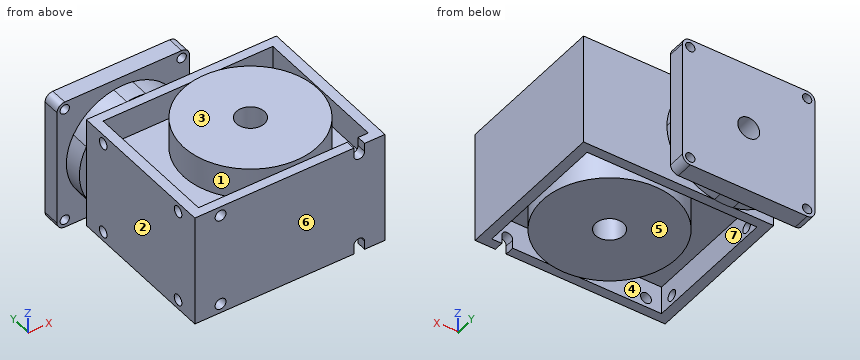
```python
from build123d import *

# Parameters (mm, degrees)
CROQUIS2_W              = 122
CROQUIS2_H              = 72
SALIENTE_EXTRUIR1_DEPTH = 100
CROQUIS3_W              = 109
CROQUIS3_H              = 88
CORTAR_EXTRUIR1_DEPTH   = 18
CROQUIS4_W              = 109
CROQUIS4_H              = 88
CORTAR_EXTRUIR2_DEPTH   = 18
SALIENTE_EXTRUIR2_DEPTH = 12
CROQUIS6_W              = 85
CROQUIS6_H              = 85
SALIENTE_EXTRUIR3_DEPTH = 11
CROQUIS7_R              = 43
SALIENTE_EXTRUIR7_DEPTH = 20
SALIENTE_EXTRUIR8_START = 20
CROQUIS8_R              = 43
SALIENTE_EXTRUIR8_DEPTH = 20
CROQUIS9_R              = 9
CORTAR_EXTRUIR3_DEPTH   = 76
CROQUIS10_R             = 3.5
CORTAR_EXTRUIR5_DEPTH   = 6
CROQUIS11_R             = 3.5
CORTAR_EXTRUIR6_DEPTH   = 6.5
CROQUIS12_R             = 7
CORTAR_EXTRUIR7_DEPTH   = 36
CROQUIS13_R             = 3
CORTAR_EXTRUIR8_DEPTH   = 11
REDONDEO2_R             = 5


with BuildPart() as part:
    # Croquis2 → Saliente-Extruir1 (new body)
    with BuildSketch(Plane(origin=(0, 0, 0), x_dir=(1, 0, 0), z_dir=(0, 1, 0))):
        Rectangle(CROQUIS2_W, CROQUIS2_H)
    extrude(amount=SALIENTE_EXTRUIR1_DEPTH)

    # Croquis3 → Cortar-Extruir1 (cut)
    with BuildSketch(Plane(origin=(0, 0, -36), x_dir=(-1, 0, 0), z_dir=(0, 0, -1))):
        with Locations((0, 50)):
            Rectangle(CROQUIS3_W, CROQUIS3_H)
    extrude(amount=-CORTAR_EXTRUIR1_DEPTH, mode=Mode.SUBTRACT)

    # Croquis4 → Cortar-Extruir2 (cut)
    with BuildSketch(Plane.XY.offset(36)):
        with Locations((0, 50)):
            Rectangle(CROQUIS4_W, CROQUIS4_H)
    extrude(amount=-CORTAR_EXTRUIR2_DEPTH, mode=Mode.SUBTRACT)

    # Croquis5 → Saliente-Extruir2 (add)
    with BuildSketch(Plane(origin=(0, 100, 0), x_dir=(1, 0, 0), z_dir=(0, 1, 0))):
        with BuildLine():
            Line((-61, 17.557049866), (-61, 0))
            Line((-61, 0), (-29, 0))
            Line((-29, 0), (7.5, 0))
            ThreePointArc((7.5, 0), (-1.143141768, 23.584856359), (-22.979202711, 36))
            Line((-22.979202711, 36), (-35.020797289, 36))
            ThreePointArc((-35.020797289, 36), (-50.128910503, 29.762713938), (-61, 17.557049866))
        make_face()
        with BuildLine():
            Line((-61, -17.557049866), (-61, 0))
            Line((-61, 0), (-61, 17.557049866))
            ThreePointArc((-61, 17.557049866), (-65.5, 0), (-61, -17.557049866))
        make_face()
        with BuildLine():
            Line((-29, 0), (-61, 0))
            Line((-61, 0), (-61, -17.557049866))
            ThreePointArc((-61, -17.557049866), (-50.128910503, -29.762713938), (-35.020797289, -36))
            Line((-35.020797289, -36), (-22.979202711, -36))
            ThreePointArc((-22.979202711, -36), (-1.143141768, -23.584856359), (7.5, 0))
            Line((7.5, 0), (-29, 0))
        make_face()
        with BuildLine():
            Line((-22.979202711, -36), (-35.020797289, -36))
            ThreePointArc((-35.020797289, -36), (-29, -36.5), (-22.979202711, -36))
        make_face()
        with BuildLine():
            ThreePointArc((-22.979202711, 36), (-29, 36.5), (-35.020797289, 36))
            Line((-35.020797289, 36), (-22.979202711, 36))
        make_face()
    extrude(amount=SALIENTE_EXTRUIR2_DEPTH)

    # Croquis6 → Saliente-Extruir3 (add)
    with BuildSketch(Plane(origin=(0, 112, 0), x_dir=(1, 0, 0), z_dir=(0, 1, 0))):
        with Locations((-29, 0)):
            Rectangle(CROQUIS6_W, CROQUIS6_H)
    extrude(amount=SALIENTE_EXTRUIR3_DEPTH)

    # Croquis7 → Saliente-Extruir7 (add)
    with BuildSketch(Plane.XY.offset(18)):
        with Locations(Location((9.5, 50, 0), (0, 0, 180))):
            Circle(CROQUIS7_R)
    extrude(amount=SALIENTE_EXTRUIR7_DEPTH)

    # Croquis8 → Saliente-Extruir8 (add)
    with BuildSketch(Plane(origin=(0, 0, -18), x_dir=(-1, 0, 0), z_dir=(0, 0, -1)).offset(SALIENTE_EXTRUIR8_START)):
        with Locations((-9.5, 50)):
            Circle(CROQUIS8_R)
    extrude(amount=-SALIENTE_EXTRUIR8_DEPTH)

    # Croquis9 → Cortar-Extruir3 (cut)
    with BuildSketch(Plane.XY.offset(38)):
        with Locations((9.5, 50)):
            Circle(CROQUIS9_R)
    extrude(amount=-CORTAR_EXTRUIR3_DEPTH, mode=Mode.SUBTRACT)

    # Croquis10 → Cortar-Extruir5 (cut)
    with BuildSketch(Plane.XZ):
        with BuildLine():
            Line((48, 36), (41, 36))
            Line((41, 36), (41, 30.5))
            ThreePointArc((41, 30.5), (44.5, 27), (48, 30.5))
            Line((48, 30.5), (48, 36))
        make_face()
        with BuildLine():
            Line((41, -30.5), (41, -36))
            Line((41, -36), (48, -36))
            Line((48, -36), (48, -30.5))
            ThreePointArc((48, -30.5), (44.5, -27), (41, -30.5))
        make_face()
        with Locations(Location((-44.5, -30, 0), (0, 0, 270))):
            Circle(CROQUIS10_R)
        with Locations(Location((-44.5, 30, 0), (0, 0, 270))):
            Circle(CROQUIS10_R)
    extrude(amount=-CORTAR_EXTRUIR5_DEPTH, mode=Mode.SUBTRACT)

    # Croquis11 → Cortar-Extruir6 (cut)
    with BuildSketch(Plane.ZY.offset(61)):
        with Locations((-30, 84.5)):
            Circle(CROQUIS11_R)
        with Locations((30, 84.5)):
            Circle(CROQUIS11_R)
        with Locations((-30, 15.5)):
            Circle(CROQUIS11_R)
        with Locations((30, 15.5)):
            Circle(CROQUIS11_R)
    extrude(amount=-CORTAR_EXTRUIR6_DEPTH, mode=Mode.SUBTRACT)

    # Croquis12 → Cortar-Extruir7 (cut)
    with BuildSketch(Plane(origin=(0, 123, 0), x_dir=(1, 0, 0), z_dir=(0, 1, 0))):
        with Locations(Location((-29, 0, 0), (0, 0, 270))):
            Circle(CROQUIS12_R)
    extrude(amount=-CORTAR_EXTRUIR7_DEPTH, mode=Mode.SUBTRACT)

    # Croquis13 → Cortar-Extruir8 (cut)
    with BuildSketch(Plane(origin=(0, 123, 0), x_dir=(1, 0, 0), z_dir=(0, 1, 0))):
        with Locations(Location((-66.5, 37.5, 0), (0, 0, 270))):
            Circle(CROQUIS13_R)
        with Locations(Location((8.5, 37.5, 0), (0, 0, 270))):
            Circle(CROQUIS13_R)
        with Locations(Location((-66.5, -37.5, 0), (0, 0, 270))):
            Circle(CROQUIS13_R)
        with Locations(Location((8.5, -37.5, 0), (0, 0, 270))):
            Circle(CROQUIS13_R)
    extrude(amount=-CORTAR_EXTRUIR8_DEPTH, mode=Mode.SUBTRACT)

    # Redondeo2
    redondeo2_edges = [part.edges().sort_by_distance(p)[0] for p in [
        (13.5, 117.5, 42.5),
        (13.5, 117.5, -42.5),
        (-71.5, 117.5, -42.5),
        (-71.5, 117.5, 42.5),
    ]]
    fillet(redondeo2_edges, radius=REDONDEO2_R)


solid = part.part
```
Read the model definition and answer for the solid it produces. Units are mm, in the model's axes. Face numbers are marked on the shaded views. A direction names the side the tool comes from. Coordinates: 2 decimals unless noted, no trailing zeros. Loops run counter-clockwise (first coordinate to the right, second up) from the corner with the lowest first, then second, coordinate; pieces in that order, holes last.
(1) The part is cut by section B-B (y = 50). Determine the outline of the cut face in (x, z), and give its area (3 significant figures).
Solution:
outline: (-61, -36) - (-54.5, -36) - (-54.5, -18) - (-33.5, -18) - (-33.5, -38) - (0.5, -38) - (0.5, 38) - (-33.5, 38) - (-33.5, 18) - (-54.5, 18) - (-54.5, 36) - (-61, 36) - close; (18.5, -38) - (52.5, -38) - (52.5, -18) - (54.5, -18) - (54.5, -36) - (61, -36) - (61, 36) - (54.5, 36) - (54.5, 18) - (52.5, 18) - (52.5, 38) - (18.5, 38) - close
area: 6,930 mm2
(2) The part is cut by section D-D (x = -44.5). Determine the outline of the cut face in (y, z).
Solution:
outline: (0, -36) - (6, -36) - (6, -33.5) - (0, -33.5) - close; (0, -26.5) - (6, -26.5) - (6, -18) - (94, -18) - (94, -36) - (100, -36) - (100, -33.05) - (112, -33.05) - (112, -42.5) - (123, -42.5) - (123, 42.5) - (112, 42.5) - (112, 33.05) - (100, 33.05) - (100, 36) - (94, 36) - (94, 18) - (6, 18) - (6, 26.5) - (0, 26.5) - close; (0, 33.5) - (6, 33.5) - (6, 36) - (0, 36) - close
(3) Flat-ended cylindrical pins translate along their axes: pin 1 Ø5.5 at (y, z) = (45.5, 25.5) entering from -X; pin 2 Ø5 at (x, z) = (-64.5, -7) entering from -Y; pin 3 Ø3 at (y, z) = (99, 7) entering from -X. Find the tip coordinate at first contact, or state that the pin passes through.
Solution:
pin 1: stops at x = -61
pin 2: stops at y = 100
pin 3: stops at x = -65.02
(4) The part is cut by section C-C (z = -22). Determine the outline of the cut face in (x, y), and give its area (3 significant figures).
Solution:
outline: (-71.5, 112) - (-58.12, 112) - (-58.12, 100) - (-61, 100) - (-61, 0) - (61, 0) - (61, 100) - (0.12, 100) - (0.12, 112) - (13.5, 112) - (13.5, 123) - (-71.5, 123) - close; circle Ø86 at (9.5, 50); hole (-54.5, 6) - (54.5, 6) - (54.5, 94) - (-54.5, 94) - close; hole circle Ø18 at (9.5, 50)
area: 9,800 mm2
(5) A tool of negligible diameter and unlimited length cuts with its end or side. For the marked faces 1, 2, 3 and 4, from which of +Z, -Z, +X, -X, +Y, -Y can it reach the whole face along a straight path? Write none if from no direction.
Solution:
face 1: +Z
face 2: +Z, -Z, -X, -Y
face 3: +Z, +X, -X, -Y
face 4: -Z
(6) The part is cut by section A-A (y = 115). Determine the outline of the cut face in (x, z), and give its area (3 significant figures).
Solution:
outline: (-71.5, -37.5) arc R5 ccw to (-66.5, -42.5) - (8.5, -42.5) arc R5 ccw to (13.5, -37.5) - (13.5, 37.5) arc R5 ccw to (8.5, 42.5) - (-66.5, 42.5) arc R5 ccw to (-71.5, 37.5) - close; hole circle Ø6 at (-66.5, -37.5); hole circle Ø6 at (-66.5, 37.5); hole circle Ø14 at (-29, 0); hole circle Ø6 at (8.5, -37.5); hole circle Ø6 at (8.5, 37.5)
area: 6,940 mm2
(7) Consider line 1 along Z through (x, y) = (-56, 84); line 2 along X through (y, z) = (120, -37); line 3 along X through (y, z) = (40, 27). Determine where each line is inside the solid, lowest interval first.
Solution:
line 1: z = -36 to -33.46, -26.54 to 26.54, 33.46 to 36
line 2: x = -71.5 to -69.46, -63.54 to 5.54, 11.46 to 13.5
line 3: x = -61 to -54.5, -32.32 to 51.32, 54.5 to 61
(8) The mould has two halves that part along Y. Classify the marked faces 5, 6 and 7: released by +Y, released by -Y, zero draft, split by the parting line, or undercut.
Solution:
face 5: zero draft
face 6: released by -Y
face 7: undercut
